Source: CAD feature listing. Evaluate the final solid. Frame: model axes, mm. A direction names the side the tool comes from. Round coordinates to 2 decimals unless told otherwise and drop trailing zeros. Loops run counter-clockwise (first coordinate to the right, second up) from the corner with the lowest first, then second, coordinate; pieces in that order, holes last. Notation, with made-up numbers: (18.5, 76.25) - (75.5, 76.25) arc R24 ccw to (75.5, 115.25) - close; hole circle Ø9 at (51.25, 26.25). An arc over 180 degrees is marked (long way). One line per question, with ' | ' between items.
from build123d import *

# Parameters (mm, degrees)
BOSS_EXTRUDE1_DEPTH = 22
BOSS_EXTRUDE2_DEPTH = 6
CUT_EXTRUDE1_DEPTH  = 6
FILLET1_R           = 0.5
SKETCH4_R           = 1.000653367
CUT_EXTRUDE2_DEPTH  = 6
SKETCH5_W           = 4.5
SKETCH5_H           = 1.5
BOSS_EXTRUDE3_DEPTH = 4.5
SKETCH7_W           = 4.5
SKETCH7_H           = 1.5
BOSS_EXTRUDE4_DEPTH = 7
SKETCH8_W           = 4.5
SKETCH8_H           = 1.5
BOSS_EXTRUDE5_DEPTH = 17
SKETCH9_R           = 1
CUT_EXTRUDE3_DEPTH  = 17
FILLET2_R           = 1
FILLET3_R           = 3
BOSS_EXTRUDE6_DEPTH = 1.5


with BuildPart() as part:
    # Sketch2 → Boss-Extrude1 (new body)
    with BuildSketch(Plane.XY):
        with BuildLine():
            Line((4.5, 5), (4.5, 0))
            ThreePointArc((4.5, 0), (5.560660172, 0.439339828), (6, 1.5))
            Line((6, 1.5), (6, 10))
            Line((6, 10), (18, 10))
            Line((18, 10), (18, 1.5))
            ThreePointArc((18, 1.5), (18.439339828, 0.439339828), (19.5, 0))
            Line((19.5, 0), (19.5, 5))
            Line((19.5, 5), (19.5, 10))
            ThreePointArc((19.5, 10), (19.060660172, 11.060660172), (18, 11.5))
            Line((18, 11.5), (6, 11.5))
            ThreePointArc((6, 11.5), (4.939339828, 11.060660172), (4.5, 10))
            Line((4.5, 10), (4.5, 5))
        make_face()
    extrude(amount=-BOSS_EXTRUDE1_DEPTH)

    # Sketch2_6 → Boss-Extrude2 (add)
    with BuildSketch(Plane.XY):
        with BuildLine():
            Line((4.5, 0), (4.5, 5))
            ThreePointArc((4.5, 5), (3.474873734, 2.525126266), (1, 1.5))
            Line((1, 1.5), (0, 1.5))
            Line((0, 1.5), (0, 0))
            Line((0, 0), (4.5, 0))
        make_face()
        with BuildLine():
            Line((23, 1.5), (24, 1.5))
            Line((24, 1.5), (24, 0))
            Line((24, 0), (19.5, 0))
            Line((19.5, 0), (19.5, 5))
            ThreePointArc((19.5, 5), (20.525126266, 2.525126266), (23, 1.5))
        make_face()
    extrude(amount=-BOSS_EXTRUDE2_DEPTH)

    # Sketch3 → Cut-Extrude1 (cut)
    with BuildSketch(Plane(origin=(0, 1.5, 0), x_dir=(1, 0, 0), z_dir=(0, 1, 0))):
        Polygon((24, 3), (24, 5.5), (19.5, 5.5), (19.5, 0.5), (24, 0.5), align=None)
        Polygon((0, 3), (0, 0.5), (4.5, 0.5), (4.5, 5.5), (0, 5.5), align=None)
    extrude(amount=CUT_EXTRUDE1_DEPTH, mode=Mode.SUBTRACT)

    # Fillet1
    fillet1_edges = [part.edges().sort_by_distance(p)[0] for p in [
        (19.5, 1.5, -3),
        (4.5, 1.5, -3),
    ]]
    fillet(fillet1_edges, radius=FILLET1_R)

    # Sketch4 → Cut-Extrude2 (cut)
    with BuildSketch(Plane(origin=(0, 1.5, 0), x_dir=(1, 0, 0), z_dir=(0, 1, 0))):
        with Locations(Location((2.25, 3, 0), (0, 0, 270))):
            Circle(SKETCH4_R)
        with Locations((21.75, 3)):
            Circle(SKETCH4_R)
    extrude(amount=-CUT_EXTRUDE2_DEPTH, mode=Mode.SUBTRACT)

    # Sketch5 → Boss-Extrude3 (add)
    with BuildSketch(Plane(origin=(0, 0, -22), x_dir=(-1, 0, 0), z_dir=(0, 0, -1))):
        with Locations((-21.75, 0.75)):
            Rectangle(SKETCH5_W, SKETCH5_H)
        with Locations((-2.25, 0.75)):
            Rectangle(SKETCH5_W, SKETCH5_H)
    extrude(amount=-BOSS_EXTRUDE3_DEPTH)

    # Sketch7 → Boss-Extrude4 (add)
    with BuildSketch(Plane(origin=(0, 0, -22), x_dir=(-1, 0, 0), z_dir=(0, 0, -1))):
        with Locations((-21.75, 0.75)):
            Rectangle(SKETCH7_W, SKETCH7_H)
        with Locations((-2.25, 0.75)):
            Rectangle(SKETCH7_W, SKETCH7_H)
    extrude(amount=BOSS_EXTRUDE4_DEPTH)

    # Sketch8 → Boss-Extrude5 (add)
    with BuildSketch(Plane(origin=(4.5, 0, 0), x_dir=(0, 0, -1), z_dir=(1, 0, 0))):
        with Locations((26.75, 0.75)):
            Rectangle(SKETCH8_W, SKETCH8_H)
    extrude(amount=BOSS_EXTRUDE5_DEPTH)

    # Sketch9 → Cut-Extrude3 (cut)
    with BuildSketch(Plane(origin=(0, 1.5, 0), x_dir=(1, 0, 0), z_dir=(0, 1, 0))):
        with Locations(Location((2.25, 26.75, 0), (0, 0, 270))):
            Circle(SKETCH9_R)
        with Locations(Location((21.75, 26.75, 0), (0, 0, 90))):
            Circle(SKETCH9_R)
    extrude(amount=-CUT_EXTRUDE3_DEPTH, mode=Mode.SUBTRACT)

    # Fillet2
    fillet2_edges = [part.edges().sort_by_distance(p)[0] for p in [
        (24, 0.75, 0),
        (0, 0.75, 0),
        (0, 0.75, -6),
        (24, 0.75, -6),
        (24, 0.75, -17.5),
        (24, 0.75, -29),
        (0, 0.75, -17.5),
        (0, 0.75, -29),
    ]]
    fillet(fillet2_edges, radius=FILLET2_R)

    # Fillet3
    fillet3_edges = [part.edges().sort_by_distance(p)[0] for p in [
        (19.5, 0.75, -17.5),
        (4.5, 0.75, -17.5),
    ]]
    fillet(fillet3_edges, radius=FILLET3_R)

    # Sketch13 → Boss-Extrude6 (add)
    with BuildSketch(Plane.XZ):
        with BuildLine():
            Line((19.5, -6), (19.5, -8))
            ThreePointArc((19.5, -8), (20.085786438, -6.585786438), (21.5, -6))
            Line((21.5, -6), (19.5, -6))
        make_face()
        with BuildLine():
            Line((4.5, -8), (4.5, -6))
            Line((4.5, -6), (2.5, -6))
            ThreePointArc((2.5, -6), (3.914213562, -6.585786438), (4.5, -8))
        make_face()
    extrude(amount=-BOSS_EXTRUDE6_DEPTH)


solid = part.part
1. Section query C-C, the plane x = 8.5. Return loops of the section in (y, z), plus the area to 4 significant figures.
Worked out:
outline: (0, -29) - (1.5, -29) - (1.5, -24.5) - (0, -24.5) - close; (10, -22) - (11.5, -22) - (11.5, 0) - (10, 0) - close | area: 39.75 mm2
2. Material intervals for probe 1 along X at (y, z) = (0.8, -26.75); probe 2 along X at (y, z) = (5, -8); probe 3 along Z at (x, y) = (21.75, 1.05), sorted ascending.
Worked out:
probe 1: x = 0 to 1.25, 3.25 to 20.75, 22.75 to 24 | probe 2: x = 4.5 to 6, 18 to 19.5 | probe 3: z = -29 to -27.75, -25.75 to -17.4, -6 to -4, -2 to 0
3. Access query for faces 1 (the flat face through (12, 1, -24.5)), 2 (the flat face through (23, 1.5, -3)), 3 (the flat face through (12, 1.5, -25)), 4 (the cylindrical face through (3.6, 0.76, -16.64)), 5 (the cylindrical face through (23.699, 0.74, -5.715)). Directions: +Z, -Z, +X, -X, +Y, -Y. A direction counts if a zero-diameter tool reaches every point of the face in a straight line with its end or side. Return the directions, or none.
Worked out:
face 1: +Y, -Y | face 2: +X, +Y | face 3: -Z, +Y | face 4: -X, +Y, -Y | face 5: +X, +Y, -Y
4. Contact query for flat-ended pins moving along their axis: P1, Ø1.6, axis at x = 3.5, z = -7, coming from the +Y side; P2, Ø4, axis at y = 2.5, z = -10.5, coming from the -X side; P3, Ø2, axis at x = 14, z = -22, coming from the -Y side. Output: stop coordinate, or through.
Worked out:
P1: stops at y = 1.5 | P2: stops at x = 4.5 | P3: stops at y = 10
5. Section query A-A, the plane y = 7.5. Return loops of the section in (x, z), plus the area to 3 significant figures.
Worked out:
outline: (4.5, -22) - (6, -22) - (6, 0) - (4.5, 0) - close; (18, -22) - (19.5, -22) - (19.5, 0) - (18, 0) - close | area: 66.0 mm2
6. Section query B-B, the plane z = -3. Return loops of the section in (x, y), plus the area to 3 significant figures.
Worked out:
outline: (0, 0) - (1.25, 0) - (1.25, 1.5) - (0, 1.5) - close; (3.25, 0) - (4.5, 0) arc R1.5 ccw to (6, 1.5) - (6, 10) - (18, 10) - (18, 1.5) arc R1.5 ccw to (19.5, 0) - (20.75, 0) - (20.75, 1.5) - (20, 1.5) arc R0.5 cw to (19.5, 2) - (19.5, 10) arc R1.5 ccw to (18, 11.5) - (6, 11.5) arc R1.5 ccw to (4.5, 10) - (4.5, 2) arc R0.5 cw to (4, 1.5) - (3.25, 1.5) - close; (22.75, 0) - (24, 0) - (24, 1.5) - (22.75, 1.5) - close | area: 58.2 mm2
7. Section query D-D, the plane z = -8.75. Return loops of the section in (x, y), plus the area to 3 significant figures.
Worked out:
outline: (4.5, 0) arc R1.5 ccw to (6, 1.5) - (6, 10) - (18, 10) - (18, 1.5) arc R1.5 ccw to (19.5, 0) - (19.5, 10) arc R1.5 ccw to (18, 11.5) - (6, 11.5) arc R1.5 ccw to (4.5, 10) - close | area: 50.6 mm2
